Check sheet for the drawn part. Datum: minimum x, y, z corner. Units: mm. A direction names the side the tool comes from. Round coordinates to 2 decimals unless told otherwise and drop trailing zeros. Loops run counter-clockwise (first coordinate to the right, second up) from the corner with the lowest first, then second, coordinate; pieces in that order, holes last. Notation, with made-up numbers: (-15, 29.25) -> (37, 29.25) arc R28 cw to (37, 67.25) -> close; hole circle Ø11 at (45.5, -15.75). An arc over 180 degrees is marked (long way). Return JSON: item names as keys, results as strings.
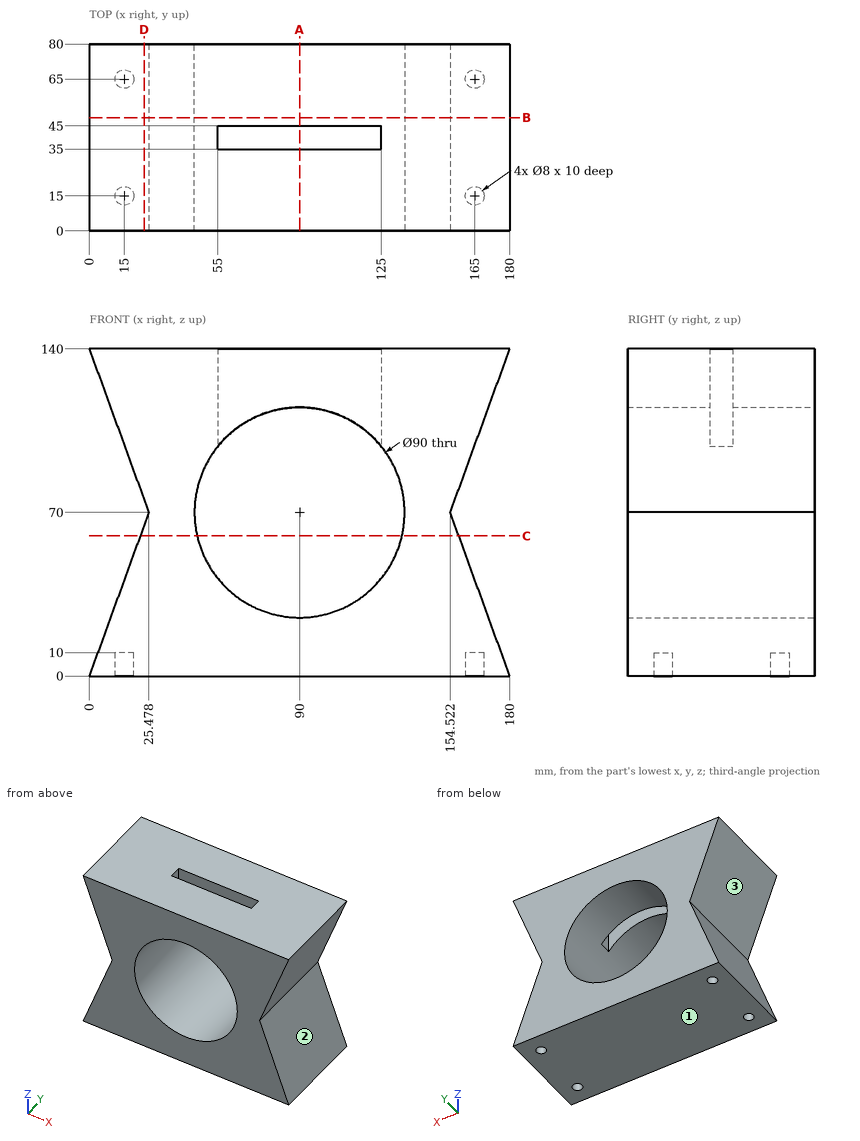
Q1. Section check A-A (x = 90). Record the boundary of the cut face in (y, z).
Results list:
{"outline": "(0, 0) -> (80, 0) -> (80, 25) -> (0, 25) -> close; (0, 115) -> (35, 115) -> (35, 140) -> (0, 140) -> close; (45, 115) -> (80, 115) -> (80, 140) -> (45, 140) -> close"}
Q2. Section check D-D (x = 23.5). Record the boundary of the cut face in (y, z).
Results list:
{"outline": "(0, 0) -> (80, 0) -> (80, 64.57) -> (0, 64.57) -> close; (0, 75.43) -> (80, 75.43) -> (80, 140) -> (0, 140) -> close"}
Q3. Material ranges on line 1 (Y direction, x = 15, z = 6); line 2 (X direction, y = 65, z = 4.25); line 3 (Z direction, x = 90, y = 45.5), recorded low to high.
Results list:
{"line 1": "0 to 11, 19 to 61, 69 to 80", "line 2": "1.55 to 11, 19 to 161, 169 to 178.45", "line 3": "0 to 25, 115 to 140"}
Q4. Go/stop test with flat-tipped pins: pin 1 (8 mm diameter, centred on x = 148, z = 31.5, fed in from -Y); pin 2 (4 mm diameter, centred on y = 39, z = 41, fed in from -X) (3 decimals); pin 3 (3 mm diameter, centred on y = 71, z = 55, fed in from +X); pin 4 (8 mm diameter, centred on y = 15.5, z = 37.5, fed in from -X). Record where each tip stops, or that it passes through.
Results list:
{"pin 1": "y = 0", "pin 2": "x = 14.195", "pin 3": "x = 160.53", "pin 4": "x = 12.19"}
Q5. Tool access check on the marked faces 1, 2 and 3. Record the directions out of +Z, -Z, +X, -X, +Y, -Y that give a thin tool (end or side, any length) a straight path to the whole face; none if there is none.
Results list:
{"face 1": "-Z, +X, -X, +Y, -Y", "face 2": "+X, +Y, -Y", "face 3": "-X, +Y, -Y"}
Q6. Section check B-B (y = 48.5). Record the boundary of the cut face in (x, z).
Results list:
{"outline": "(0, 0) -> (180, 0) -> (154.52, 70) -> (180, 140) -> (0, 140) -> (25.48, 70) -> close; hole circle Ø90 at (90, 70)"}
Q7. Section check C-C (z = 60). Record the boundary of the cut face in (x, y), then the cut area to 3 significant figures.
Results list:
{"outline": "(21.84, 0) -> (46.13, 0) -> (46.13, 80) -> (21.84, 80) -> close; (133.87, 0) -> (158.16, 0) -> (158.16, 80) -> (133.87, 80) -> close", "area": "3,890 mm^2"}
